```python
from build123d import *

# Parameters (mm, degrees)
MODEL_W             = 20.32
MODEL_H             = 17.78
MODEL_R             = 1.524
MODEL_W_2           = 6.1999876
MODEL_H_2           = 6.3999872
BOSS_EXTRUDE1_DEPTH = 2
MODEL_3_W           = 6.1999876
MODEL_3_H           = 6.3999872
BOSS_EXTRUDE2_DEPTH = 10
FILLET1_R           = 2


with BuildPart() as part:
    # Model → Boss-Extrude1 (new body)
    with BuildSketch(Plane.XY):
        with Locations((10.16, 8.89)):
            Rectangle(MODEL_W, MODEL_H)
        with Locations((2.54, 7.62)):
            Circle(MODEL_R, mode=Mode.SUBTRACT)
        with Locations((17.78, 15.24)):
            Circle(MODEL_R, mode=Mode.SUBTRACT)
        with Locations((10.16, 11.43)):
            Rectangle(MODEL_W_2, MODEL_H_2, mode=Mode.SUBTRACT)
    extrude(amount=BOSS_EXTRUDE1_DEPTH)

    # Model<3> → Boss-Extrude2 (add)
    with BuildSketch(Plane.XY):
        with Locations((10.16, 11.43)):
            Rectangle(MODEL_3_W, MODEL_3_H)
    extrude(amount=BOSS_EXTRUDE2_DEPTH)

    # Fillet1
    fillet1_edges = [part.edges().sort_by_distance(p)[0] for p in [
        (7.0600062, 14.6299936, 6),
        (7.0600062, 8.2300064, 6),
        (13.2599938, 8.2300064, 6),
        (13.2599938, 14.6299936, 6),
    ]]
    fillet(fillet1_edges, radius=FILLET1_R)


solid = part.part
```
Input: part model. Units: mm. Frame: model coordinates. A direction names the side the tool comes from. Round coordinates to 2 decimals unless told otherwise and drop trailing zeros. Write each loop counter-clockwise with the first axis right and the second up, starting at its lowest first coordinate (ties: lowest second). Pieces come first, ordered by that corner, then holes. Notation, with made-up numbers: (8.25, -6) - (26.25, -6) arc R28 ccw to (26.25, 30) - close; hole circle Ø7 at (-11.5, -14.75). An arc over 180 degrees is marked (long way). Write item = value, one per line.
(1) Access query for faces 4 (the flat face through (10, 14.63, 6)), 5 (the cylindrical face through (12.66, 8.8, 6.06)), 6 (the flat face through (7.06, 11, 6)), 7 (the cylindrical face through (7.63, 14.03, 6.06)). Directions: +Z, -Z, +X, -X, +Y, -Y. A direction counts if a zero-diameter tool reaches every point of the face in a straight line with its end or side. Return the directions, or none.
Geometry check:
face_4 = +Z, +X, -X, +Y
face_5 = +Z, +X, -Y
face_6 = +Z, -X, +Y, -Y
face_7 = +Z, -X, +Y
(2) Section query A-A on x = 17.78. Output: boundary loops of the cut face in (y, z).
Geometry check:
outline = (0, 0) - (13.72, 0) - (13.72, 2) - (0, 2) - close; (16.76, 0) - (17.78, 0) - (17.78, 2) - (16.76, 2) - close
(3) Pull-direction query (Y, two-part tool) for faces 1 (the flat face through (10, 8.23, 6)), 2 (the cylindrical face through (2.21, 6.132, 0.986)), 3 (the flat face through (13.26, 11, 6)); classes: +Y half, -Y half, draft (parallel to the pull), parting line (faces both ways), or undercut.
Geometry check:
face_1 = -Y half
face_2 = undercut
face_3 = draft
(4) Contact query for flat-ended pins moving along their axis: pin 1 Ø1.5 at (y, z) = (9, 6.5) entering from +X; pin 2 Ø9 at (x, y) = (6.5, 13) entering from +Z; pin 3 Ø3 at (y, z) = (10, 5.5) entering from +X; pin 4 Ø1.1 at (x, z) = (9.5, 7) entering from -Y. Output: stop coordinate, or through.
Geometry check:
pin_1 = 13.2
pin_2 = 10
pin_3 = 13.26
pin_4 = 8.23
(5) Material intervals for probe 1 along Y at (x, z) = (2.54, 1.65); probe 2 along Z at (x, y) = (19, 7.25); probe 3 along X at (y, z) = (11, 5), sorted ascending.
Geometry check:
probe_1 = 0 to 6.1, 9.14 to 17.78
probe_2 = 0 to 2
probe_3 = 7.06 to 13.26
(6) Section query D-D on z = 4. Output: boundary loops of the cut face in (x, y), then the cut area to 3 significant figures.
Geometry check:
outline = (7.06, 10.23) arc R2 ccw to (9.06, 8.23) - (11.26, 8.23) arc R2 ccw to (13.26, 10.23) - (13.26, 12.63) arc R2 ccw to (11.26, 14.63) - (9.06, 14.63) arc R2 ccw to (7.06, 12.63) - close
area = 36.2 mm^2
(7) Section query B-B on y = 15.24. Output: boundary loops of the cut face in (x, z), then the cut area to 3 significant figures.
Geometry check:
outline = (0, 0) - (16.26, 0) - (16.26, 2) - (0, 2) - close; (19.3, 0) - (20.32, 0) - (20.32, 2) - (19.3, 2) - close
area = 34.5 mm^2
(8) Section query C-C on z = 1.25. Output: boundary loops of the cut face in (x, y).
Geometry check:
outline = (0, 0) - (20.32, 0) - (20.32, 17.78) - (0, 17.78) - close; hole circle Ø3.05 at (2.54, 7.62); hole circle Ø3.05 at (17.78, 15.24)
